Autodesk Inventor part; units mm, degrees
ref_plane "YZ Plane" through (0, 0, 0) normal (1, 0, 0) x (0, 1, 0)
ref_plane "XZ Plane" through (0, 0, 0) normal (0, 1, 0) x (-1, 0, 0)
ref_plane "XY Plane" through (0, 0, 0) normal (0, 0, 1) x (1, 0, 0)
sketch "Sketch1" plane through (0, 0, 0) normal (0, 0, 1) x (1, 0, 0)
  circle A0 centre (-24.464, 35.97) radius 1.27
  circle A1 centre (31.416, 0) radius 3.175
  line L0 (-56.214, -50.8) -> (-56.214, 50.8)
  line L1 (97.7735, -50.8) -> (-56.214, -50.8)
  line L2 (97.7735, 50.8) -> (97.7735, -50.8)
  line L3 (-56.214, 50.8) -> (97.7735, 50.8)
  circle A2 centre (9.7431, -32.1205) radius 12.7
  circle A3 centre (-24.464, 35.97) radius 12.7
  circle A4 centre (31.416, 0) radius 11.4366
  line L4 (111.6872, -61.5577) -> (-85.1628, -61.5577)
  line L5 (-85.1628, -61.5577) -> (-85.1628, 90.8423)
  line L6 (-85.1628, 90.8423) -> (111.6872, 90.8423)
  line L7 (111.6872, 90.8423) -> (111.6872, -61.5577)
  point P0 (0, 0)
  dimension "d0" = 196.85
  dimension "d1" = 152.4
extrude "Extrusion1" add sketch "Sketch1" along normal blind 6.35 contours L0 L3 L2 L1 | L4 L5 L6 L7
properties part number "tiltBoxBase"
The model under review builds one solid part; all positions refer to its coordinate system, in mm. Coordinates: 2 decimals unless noted, no trailing zeros. Loops run counter-clockwise (first coordinate to the right, second up) from the corner with the lowest first, then second, coordinate; pieces in that order, holes last.
(1) Wall thickness on L1, parallel to X at y = 37, z = 5.25; L2, parallel to X at y = 34, z = 1.5; L3, parallel to Y at x = 23.5, z = 4.75: over which ranges is each line inside the solid? List them lowest first.
Determined:
L1: x = -85.16 to -37.12, -11.81 to 111.69
L2: x = -85.16 to -37.01, -11.92 to 111.69
L3: y = -61.56 to -8.25, 8.25 to 90.84
(2) Draft analysis for pull direction X (two halves, no side actions). For faces 1 (the flat face through (12, 90.842, 3)), 2 (the flat face through (111.687, 16, 3)), 3 (the cylindrical face through (-33.824, 27.387, 3.131)), 4 (the flat face through (-85.163, 14, 3)), state which applies: +X half, -X half, draft (parallel to the pull), parting line (faces both ways), or undercut.
Determined:
face 1: draft
face 2: +X half
face 3: undercut
face 4: -X half
(3) Consider section C-C, the plane z = 2.5. Give the boundary of the cut face in (x, y), plus the area to 3 significant figures.
Determined:
outline: (-85.16, -61.56) - (111.69, -61.56) - (111.69, 90.84) - (-85.16, 90.84) - close; hole circle Ø25.4 at (-24.46, 35.97); hole circle Ø25.4 at (9.74, -32.12); hole circle Ø22.87 at (31.42, 0)
area: 28,600 mm2
(4) Consider section B-B, the plane x = -22.5. Give the boundary of the cut face in (y, z).
Determined:
outline: (-61.56, 0) - (23.42, 0) - (23.42, 6.35) - (-61.56, 6.35) - close; (48.52, 0) - (90.84, 0) - (90.84, 6.35) - (48.52, 6.35) - close
(5) Insertion check: P1, Ø5, axis at x = 15, y = 17.5, coming from the -Z side. The pin has a flat end and moves straight along its axis. Give the tip position at first contact, or say it passes through.
Determined:
P1: stops at z = 0
(6) Consider section A-A, the plane y = 0. Give the boundary of the cut face in (x, z), plus the area to 3 significant figures.
Determined:
outline: (-85.16, 0) - (19.98, 0) - (19.98, 6.35) - (-85.16, 6.35) - close; (42.85, 0) - (111.69, 0) - (111.69, 6.35) - (42.85, 6.35) - close
area: 1,100 mm2
